```python
from build123d import *

# Parameters (mm, degrees)
EXTRUDE_THIN1_DEPTH = 381
FILLET1_R           = 1.27


with BuildPart() as part:
    # Sketch1 → Extrude-Thin1 (new body)
    with BuildSketch(Plane.XY):
        with BuildLine():
            Line((-17.4625, 0), (-23.8125, 0))
            Line((-23.8125, 0), (-23.8125, 7.9375))
            Line((-23.8125, 7.9375), (-22.225, 7.9375))
            ThreePointArc((-22.225, 7.9375), (-19.202708098, 15.233958098), (-11.90625, 18.25625))
            Line((-11.90625, 18.25625), (-11.90625, 24.60625))
            ThreePointArc((-11.90625, 24.60625), (-7.977387947, 26.233637947), (-6.35, 30.1625))
            Line((-6.35, 30.1625), (-6.35, 38.1))
            Line((-6.35, 38.1), (0, 38.1))
            Line((0, 38.1), (0, 34.925))
            Line((0, 34.925), (-1.27, 34.925))
            Line((-1.27, 34.925), (-1.27, 36.83))
            Line((-1.27, 36.83), (-5.08, 36.83))
            Line((-5.08, 36.83), (-5.08, 30.1625))
            ThreePointArc((-5.08, 30.1625), (-6.649491181, 25.807712315), (-10.63625, 23.45542992))
            Line((-10.63625, 23.45542992), (-10.63625, 16.896683923))
            ThreePointArc((-10.63625, 16.896683923), (-18.304682486, 14.335932486), (-20.865433923, 6.6675))
            Line((-20.865433923, 6.6675), (-22.5425, 6.6675))
            Line((-22.5425, 6.6675), (-22.5425, 1.27))
            Line((-22.5425, 1.27), (-17.4625, 1.27))
            Line((-17.4625, 1.27), (-17.4625, 0))
        make_face()
    extrude(amount=-EXTRUDE_THIN1_DEPTH)

    # Fillet1
    fillet1_edges = [part.edges().sort_by_distance(p)[0] for p in [
        (-10.63625, 16.896683923, -190.5),
        (-20.865433923, 6.6675, -190.5),
        (-23.8125, 0, -190.5),
        (-23.8125, 7.9375, -190.5),
        (-11.90625, 24.60625, -190.5),
        (-6.35, 38.1, -190.5),
        (0, 38.1, -190.5),
    ]]
    fillet(fillet1_edges, radius=FILLET1_R)


solid = part.part
```
Input: part model. Units: mm. Frame: model coordinates. A direction names the side the tool comes from. Coordinates: 2 decimals unless noted, no trailing zeros. Use one line per item in the form item = value.
Q1. Draft query along Y for faces 1 (the face through (-6.608, 25.859, -187.833)), 2 (the face through (-19.282, 15.153, -187.833)), 3 (the face through (-18.23, 14.41, -187.83)), 4 (the face through (-5.08, 34, -188)). Return one class per face: released by +Y, released by -Y, zero draft, split by the parting line, or undercut.
Answer below:
face_1 = released by -Y
face_2 = released by +Y
face_3 = undercut
face_4 = zero draft
Q2. Material intervals for probe 1 along Y at (x, z) = (-3, -225); probe 2 along X at (y, z) = (30, -251); probe 3 along X at (y, z) = (20.5, -20.5), sorted ascending. Write a range as from..to.
Answer below:
probe_1 = 36.83..38.1
probe_2 = -6.35..-5.08
probe_3 = -11.91..-10.64
Q3. Set-up query: faces 5 (the face through (-11, 19, -381)), 6 (the face through (-6.35, 33, -188)). Return all of +Z, -Z, +X, -X, +Y, -Y with unobstructed straight access to the full face (end or side cutting, diameter ignored); none if empty.
Answer below:
face_5 = -Z, +X, -X, +Y, -Y
face_6 = +Z, -Z, -X, +Y
Q4. First-contact query: pin 1 (1 mm diameter, centred on x = -1, z = -245.5, fed in from -Y) (3 decimals); pin 2 (4 mm diameter, centred on y = 28.5, z = -188, fed in from -X); pin 3 (4.5 mm diameter, centred on y = 3, z = -144, fed in from +X). Flat tips, straight axial feed; report the tip coordinate or a pass-through.
Answer below:
pin_1 = 34.925
pin_2 = -7.73
pin_3 = -17.46
